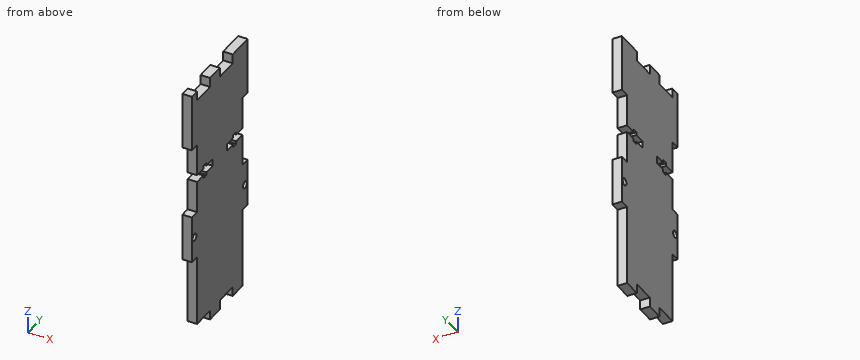
Autodesk Inventor part; units mm, degrees
ref_plane "YZ Plane" through (0, 0, 0) normal (1, 0, 0) x (0, 1, 0)
ref_plane "XZ Plane" through (0, 0, 0) normal (0, 1, 0) x (-1, 0, 0)
ref_plane "XY Plane" through (0, 0, 0) normal (0, 0, 1) x (1, 0, 0)
sketch "Sketch1" plane through (0, 0, 0) normal (1, 0, 0) x (0, 1, 0)
  line L0 (-17.5, 50) -> (17.5, 50)
  line L1 (17.5, 50) -> (17.5, -50)
  line L2 (17.5, -50) -> (-17.5, -50)
  line L3 (-17.5, -50) -> (-17.5, 50)
  line L4 (-17.5, 50) -> (17.5, -50) construction
  line L5 (17.5, 50) -> (-17.5, -50) construction
  line L6 (17.5, 50) -> (10, 50)
  line L7 (10, 50) -> (10, 54)
  line L8 (10, 54) -> (17.5, 54)
  line L9 (17.5, 54) -> (17.5, 50)
  line L10 (0, 50) -> (-7.5, 50)
  line L11 (-7.5, 50) -> (-7.5, 54)
  line L12 (-7.5, 54) -> (0, 54)
  line L13 (0, 54) -> (0, 50)
  line L14 (17.5, 0) -> (-17.5, 0) construction
  line L15 (0, 50) -> (0, -50) construction
  line L16 (17.5, -50) -> (10, -50)
  line L17 (10, -50) -> (10, -54)
  line L18 (10, -54) -> (17.5, -54)
  line L19 (17.5, -54) -> (17.5, -50)
  line L20 (0, -50) -> (-7.5, -50)
  line L21 (-7.5, -50) -> (-7.5, -54)
  line L22 (-7.5, -54) -> (0, -54)
  line L23 (0, -54) -> (0, -50)
  line L24 (17.5, 50) -> (21.5, 50)
  line L25 (21.5, 50) -> (21.5, 30)
  line L26 (21.5, 30) -> (17.5, 30)
  line L27 (17.5, 30) -> (17.5, 50)
  line L28 (17.5, 0) -> (21.5, 0)
  line L29 (21.5, 0) -> (21.5, -20)
  line L30 (21.5, -20) -> (17.5, -20)
  line L31 (17.5, -20) -> (17.5, 0)
  line L32 (-17.5, 0) -> (-21.5, 0)
  line L33 (-21.5, 0) -> (-21.5, -20)
  line L34 (-21.5, -20) -> (-17.5, -20)
  line L35 (-17.5, -20) -> (-17.5, 0)
  line L36 (17.5, 50) -> (21.5, 50)
  line L37 (21.5, 50) -> (21.5, 54)
  line L38 (21.5, 54) -> (17.5, 54)
  line L39 (17.5, 54) -> (17.5, 50)
  line L40 (-17.5, 30) -> (-21.5, 30)
  line L41 (-21.5, 30) -> (-21.5, 54)
  line L42 (-21.5, 54) -> (-17.5, 54)
  line L43 (-17.5, 54) -> (-17.5, 30)
  point P0 (0, 0)
  point P1 (0, 52)
  point P2 (0, -52)
  point P3 (-17.5, -20)
  point P4 (-7.5, -50)
  point P5 (10, -50)
  point P6 (17.5, -20)
  point P7 (17.5, 30)
  point P8 (10, 50)
  point P9 (-7.5, 50)
  point P10 (-19.5, 0)
  point P11 (-19.5, 30)
  dimension "d0" = 35
  dimension "d2" = 7.5
  dimension "d3" = 4
  dimension "d4" = 7.5
  dimension "d5" = 4
  dimension "d6" = 10
  dimension "d7" = 4
  dimension "d8" = 20
  dimension "d9" = 4
  dimension "d10" = 20
  dimension "d13" = 4
  dimension "d14" = 20
  dimension "d17" = 4
  dimension "d18" = 24
  dimension "d19" = 30
extrude "Extrusion1" add sketch "Sketch1" along normal blind 4
sketch "Sketch2" plane through (0, 0, 0) normal (-1, 0, 0) x (0, 0, 1)
  line L0 (-8.5, 17.5) -> (-11.5, 17.5) construction
  line L1 (-8.5, 21.5) -> (-8.5, 17.5) construction
  line L2 (-11.5, 21.5) -> (-8.5, 21.5) construction
  line L3 (-11.5, 21.5) -> (-11.5, 17.5) construction
  line L4 (13.5, 21.5) -> (16.5, 21.5)
  line L5 (-11.5, 21.5) -> (-8.5, 17.5) construction
  circle A0 centre (-10, 19.5) radius 1.5
  line L6 (13.5, 17.5) -> (16.5, 17.5)
  line L7 (16.5, 17.5) -> (16.5, 5.5)
  line L8 (16.5, 5.5) -> (13.5, 5.5)
  line L9 (13.5, 5.5) -> (13.5, 17.5)
  line L10 (0, 17.5) -> (30, 17.5)
  line L11 (12.3, 10.3) -> (17.7, 10.3)
  line L12 (17.7, 10.3) -> (17.7, 12.7)
  line L13 (17.7, 12.7) -> (12.3, 12.7)
  line L14 (12.3, 12.7) -> (12.3, 10.3)
  line L15 (13.5, -5.5) -> (16.5, -5.5)
  line L16 (16.5, -5.5) -> (16.5, -17.5)
  line L17 (16.5, -17.5) -> (13.5, -17.5)
  line L18 (13.5, -17.5) -> (13.5, -5.5)
  line L19 (12.3, -12.7) -> (17.7, -12.7)
  line L20 (17.7, -12.7) -> (17.7, -10.3)
  line L21 (17.7, -10.3) -> (12.3, -10.3)
  line L22 (12.3, -10.3) -> (12.3, -12.7)
  line L23 (30, -17.5) -> (0, -17.5)
  line L24 (16.5, -21.5) -> (13.5, -21.5)
  line L25 (30, 21.5) -> (54, 21.5) construction
  line L26 (54, 21.5) -> (54, 10) construction
  line L27 (54, 10) -> (50, 10) construction
  line L28 (50, 10) -> (50, 0) construction
  line L29 (50, 0) -> (54, 0) construction
  line L30 (54, 0) -> (54, -7.5) construction
  line L31 (54, -7.5) -> (50, -7.5) construction
  line L32 (50, -7.5) -> (50, -17.5) construction
  line L33 (50, -17.5) -> (54, -17.5) construction
  line L34 (54, -17.5) -> (54, -21.5) construction
  line L35 (54, -21.5) -> (30, -21.5) construction
  line L36 (30, -21.5) -> (30, -17.5) construction
  line L37 (30, -17.5) -> (0, -17.5) construction
  line L38 (0, -17.5) -> (0, -21.5) construction
  line L39 (0, -21.5) -> (-20, -21.5) construction
  line L40 (-20, -21.5) -> (-20, -17.5) construction
  line L41 (-20, -17.5) -> (-50, -17.5) construction
  line L42 (-50, -17.5) -> (-50, -7.5) construction
  line L43 (-50, -7.5) -> (-54, -7.5) construction
  line L44 (-54, -7.5) -> (-54, 0) construction
  line L45 (-54, 0) -> (-50, 0) construction
  line L46 (-50, 0) -> (-50, 10) construction
  line L47 (-50, 10) -> (-54, 10) construction
  line L48 (-54, 10) -> (-54, 17.5) construction
  line L49 (-54, 17.5) -> (-20, 17.5) construction
  line L50 (-20, 17.5) -> (-20, 21.5) construction
  line L51 (-20, 21.5) -> (0, 21.5) construction
  line L52 (0, 21.5) -> (0, 17.5) construction
  line L53 (0, 17.5) -> (30, 17.5) construction
  line L54 (30, 17.5) -> (30, 21.5) construction
  line L55 (-11.5, -17.5) -> (-8.5, -17.5) construction
  line L56 (-11.5, -21.5) -> (-11.5, -17.5) construction
  line L57 (-8.5, -21.5) -> (-11.5, -21.5) construction
  line L58 (-8.5, -21.5) -> (-8.5, -17.5) construction
  line L59 (-11.5, -17.5) -> (-8.5, -21.5) construction
  circle A1 centre (-10, -19.5) radius 1.5
  point P0 (0, 0)
  point P1 (15, 17.5)
  point P2 (15, 21.5)
  point P3 (15, 12.7)
  point P4 (17.7, 11.5)
  point P5 (16.5, 11.5)
  point P6 (15, -5.5)
  point P7 (15, -10.3)
  point P8 (17.7, -11.5)
  point P9 (16.5, -11.5)
  point P10 (15, -21.5)
  point P11 (16.5, 12.7)
  point P12 (13.5, 12.7)
  point P13 (13.5, 10.3)
  point P14 (16.5, 10.3)
  point P15 (13.5, -10.3)
  point P16 (13.5, -12.7)
  point P17 (16.5, -12.7)
  point P18 (16.5, -10.3)
  dimension "d20" = 3
  dimension "d21" = 3
  dimension "d22" = 12
  dimension "d23" = 5.4
  dimension "d24" = 2.4
  dimension "d25" = 3
  dimension "d26" = 12
  dimension "d27" = 5.4
  dimension "d28" = 2.4
  dimension "d31" = 3
extrude "Extrusion2" cut sketch "Sketch2" against normal up to next
properties part number "FloorButtonHolder_Side_V1" material "MDF Medium Density Fiberboard"
Design review of the part built by this model. Coordinates are the model's own, in mm. Round coordinates to 2 decimals unless told otherwise and drop trailing zeros. Order: outer loops, then holes, each group sorted by start corner. A loop starts at its lowest first (then second) coordinate and runs counter-clockwise, first axis right, second up. Notation, with made-up numbers: M -19.5,72 L 0.5,72 A15 cw 0.5,90 Z; hole C -11.75,85 d5. An arc over 180 degrees is marked long. Answer as CSV lines item,"result". Start each with the question number.
1) For pin 1 Ø0.6 at (x, z) = (3, 12.5) entering from -Y; pin 2 Ø6 at (y, z) = (15, -9) entering from -X; pin 3 Ø2 at (x, y) = (1, 19.5) entering from -Z, all flat-tipped, find the tip position at first contact; note any pin that passes through.
2) Add section A-A (z = -10). Give the boundary of the cut face in (x, y).
3) Add section C-C (y = 7). Give the boundary of the cut face in (x, z).
4) Add section D-D (x = 2.75). Give the number of separate pieces and of enclosed holes in the cut face, then the cut area to 3 significant figures.
5) Wall thickness on line 1 along Y through (x, z) = (0.9, -10); line 2 along Z through (x, y) = (0.8, 8); line 3 along Z through (x, y) = (2.1, -7): over which ranges is each line inside the solid? List them lowest first. Write a range as [from, to].
6) Add section B-B (y = -19.5). Give the boundary of the cut face in (x, z), then the cut area to 3 significant figures.
Resolved:
1,pin 1,"y = -17.5"
1,pin 2,"x = 0"
1,pin 3,"z = -20"
2,outline,"M 0,-21.5 L 4,-21.5 L 4,-21 L 0,-21 Z; M 0,-18 L 4,-18 L 4,18 L 0,18 Z; M 0,21 L 4,21 L 4,21.5 L 0,21.5 Z"
3,outline,"M 0,-50 L 4,-50 L 4,13.5 L 0,13.5 Z; M 0,16.5 L 4,16.5 L 4,50 L 0,50 Z"
4,separate pieces,"1"
4,enclosed holes,"2"
4,area,"3,870 mm^2"
5,line 1,"[-21.5, -21], [-18, 18], [21, 21.5]"
5,line 2,"[-50, 13.5], [16.5, 50]"
5,line 3,"[-54, 13.5], [16.5, 54]"
6,outline,"M 0,-20 L 4,-20 L 4,-11.5 L 0,-11.5 Z; M 0,-8.5 L 4,-8.5 L 4,0 L 0,0 Z; M 0,30 L 4,30 L 4,54 L 0,54 Z"
6,area,"164 mm^2"
